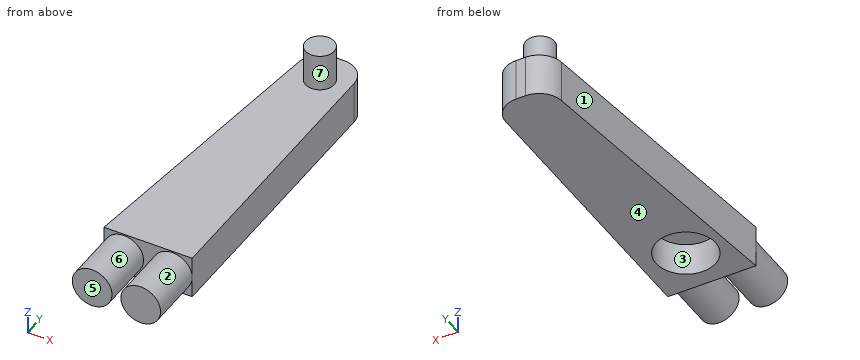
Autodesk Inventor part; units mm, degrees
ref_plane "YZ Plane" through (0, 0, 0) normal (1, 0, 0) x (0, 1, 0)
ref_plane "XZ Plane" through (0, 0, 0) normal (0, 1, 0) x (-1, 0, 0)
ref_plane "XY Plane" through (0, 0, 0) normal (0, 0, 1) x (1, 0, 0)
sketch "Sketch1" plane through (0, 0, 0) normal (0, 0, 1) x (1, 0, 0)
  circle A0 centre (0, 0) radius 38.1
  line L0 (-56.515, -58.42) -> (56.515, -58.42)
  line L1 (56.515, -58.42) -> (56.515, 335.28)
  line L2 (56.515, 335.28) -> (-13.335, 335.28)
  line L3 (-13.335, 335.28) -> (-56.515, -58.42)
  dimension "d0" = 76.2
  dimension "d1" = 393.7
  dimension "d2" = 113.03
  dimension "d3" = 69.85
  dimension "d4" = 58.42
  dimension "d5" = 56.515
extrude "Extrusion1" add sketch "Sketch1" against normal blind 54.3243
fillet "Fillet1" radius 30.48 2 edges at (56.515, 335.28, -27.1621) (-13.335, 335.28, -27.1621)
sketch "Sketch2" plane through (-56.515, -58.42, 0) normal (0, -1, 0) x (1, 0, 0)
  line L0 (113.03, 0) -> (113.03, -54.3243)
  line L1 (113.03, -27.1621) -> (0, -27.1621)
  line L2 (0, 0) -> (0, -54.3243)
  line L3 (56.515, -27.1621) -> (56.515, -44.3071)
  circle A0 centre (87.63, -27.1621) radius 25.4
  circle A1 centre (25.4, -27.1621) radius 25.4
  point P0 (56.515, 0)
  dimension "d10" = 50.8
  dimension "d9" = 50.8
  dimension "d11" = 113.03
extrude "Extrusion2" add sketch "Sketch2" along normal blind 71.12
sketch "Sketch3" plane through (0, 0, 0) normal (0, 0, 1) x (1, 0, 0)
  circle A0 centre (0, 0) radius 42.7153
extrude "Extrusion3" add sketch "Sketch3" against normal blind 12.7
sketch "Sketch4" plane through (0, 0, -54.3243) normal (0, 0, -1) x (-1, 0, 0)
  line L0 (-26.035, 335.28) -> (-13.9848, 335.28)
  line L1 (-20.0099, 335.28) -> (-20.0099, 292.1)
  circle A0 centre (-20.0099, 292.1) radius 18.415
  point P0 (0, 0)
  dimension "d17" = 36.83
  dimension "d20" = 292.1
extrude "Extrusion4" add sketch "Sketch4" against normal blind 101.6
equation "\"d10\" = d9"
properties part number "Forearm-lrg"
The model under review builds one solid part; all positions refer to its coordinate system, in mm. Face numbers are marked on the shaded views. A direction names the side the tool comes from. Give positions to 0.01 mm unless a question says otherwise; leave off trailing zeros. Write each loop counter-clockwise with the first axis right and the second up, starting at its lowest first coordinate (ties: lowest second). Pieces come first, ordered by that corner, then holes.
(1) Consider section C-C, the plane z = 12. Give the boundary of the cut face in (x, y) (3 decimals).
(2) The part is to be moulded in two halves that separate along X. For the marked faces 1, 2, 3 and 4, say which applies: released by +X, released by -X, zero draft, split by the parting line, or undercut.
(3) To check wall thickness, follow L1, parallel to Z at x = -21.5, y = -25; L2, parallel to Z at x = -10.5, y = 121.5; L3, parallel to Y at x = 0, z = -38. State the ranges of each line that lie inside material, in increasing order.
(4) For P1, Ø1, axis at x = 28, y = 232.5, coming from the +Z side; P2, Ø23, axis at x = 5.5, y = 14.5, coming from the -Z side; P3, Ø12, axis at x = 37.5, z = -34.5, coming from the +Y side, all flat-tipped, find the tip position at first contact; note any pin that passes through.
(5) Consider section B-B, the plane x = 22. Give the boundary of the cut face in (y, z).
(6) Consider section D-D, the plane y = -75. Give the boundary of the cut face in (x, z) (3 decimals).
(7) Consider section A-A, the plane y = 292.1. Give the boundary of the cut face in (x, z) (3 decimals).
(8) Tool access review of the marked faces 5, 6 and 7: name each direction out of +Z, -Z, +X, -X, +Y, -Y from which nothing blocks a thin tool from reaching the whole face with its end or side.
Returned:
1. outline: circle Ø36.83 at (20.01, 292.1)
2. face 1: released by -X
2. face 2: undercut
2. face 3: undercut
2. face 4: zero draft
3. L1: z = -12.7 to 0
3. L2: z = -54.32 to 0
3. L3: y = -58.42 to -38.1, 38.1 to 331.88
4. P1: stops at z = 0
4. P2: stops at z = -12.7
4. P3: stops at y = 334.79
5. outline: (-129.54, -50.87) - (-58.42, -50.87) - (-58.42, -54.32) - (-31.11, -54.32) - (-31.11, -12.7) - (31.11, -12.7) - (31.11, -54.32) - (335.28, -54.32) - (335.28, 0) - (310.41, 0) - (310.41, 47.28) - (273.79, 47.28) - (273.79, 0) - (-58.42, 0) - (-58.42, -3.45) - (-129.54, -3.45) - close
6. outline: circle Ø50.8 at (-31.115, -27.162); circle Ø50.8 at (31.115, -27.162)
7. outline: (-18.071, -54.324) - (56.515, -54.324) - (56.515, 0) - (38.425, 0) - (38.425, 47.276) - (1.595, 47.276) - (1.595, 0) - (-18.071, 0) - close
8. face 5: +Z, -Z, +X, -X, -Y
8. face 6: -Y
8. face 7: +Z
